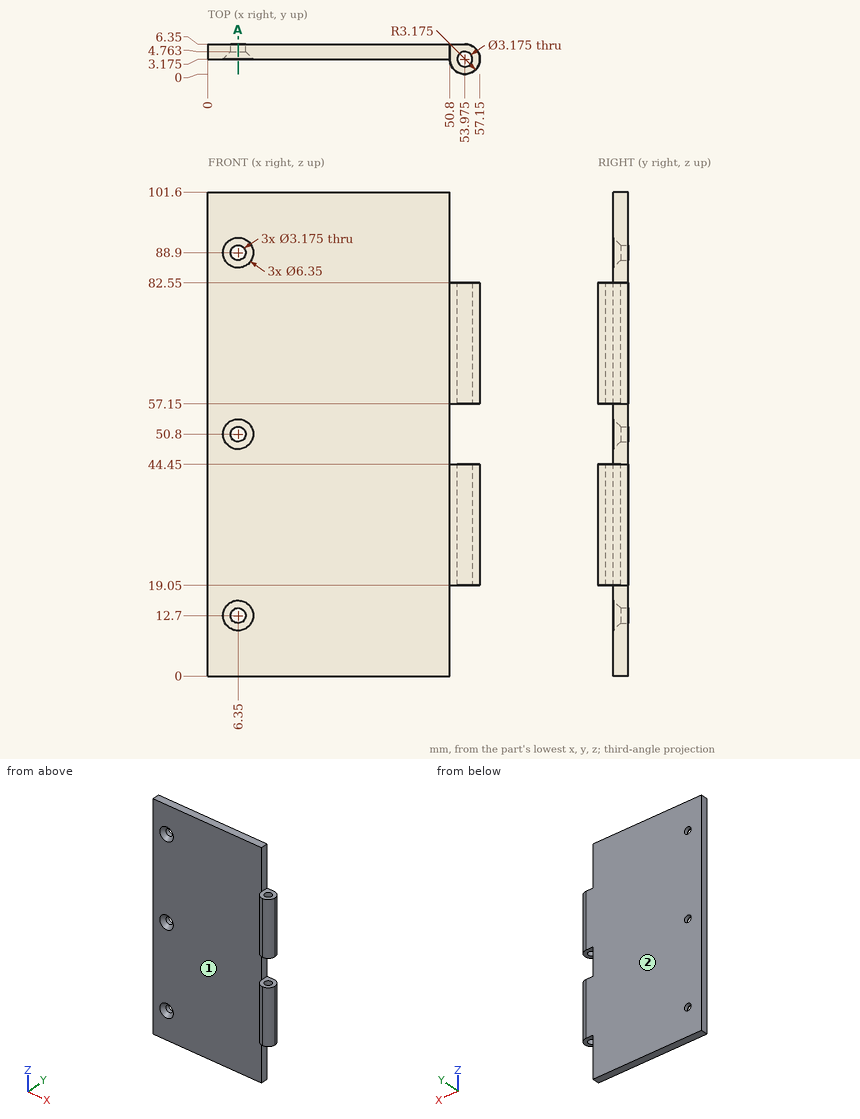
Geometry: see drawing. Coordinates: mm, zero at the bounding-box minimum. A direction names the side the tool comes from. Round coordinates to 2 decimals unless told otherwise and drop trailing zeros. Write item = value, one per line. Start each with the question number.
(1) Set-up query: the marked faces 1 and 2. Return all of +Z, -Z, +X, -X, +Y, -Y with unobstructed straight access to the full face (end or side cutting, diameter ignored); none if empty.
(2) Section query A-A, the plane x = 6.35. State how many separate pieces and enclosed holes the cut face has, plus the area to 3 significant figures.
(3) Pin query (flat end, axial travel): pin 1 (2.5 mm diameter, centred on x = 6.35, z = 88.9, fed in from +Y); pin 2 (8 mm diameter, centred on x = 29, z = 38.5, fed in from -Y) (1 decimal); pin 3 (3 mm diameter, centred on x = 54, y = 3.5, fed in from +Z); pin 4 (3.5 mm diameter, centred on y = 4.5, z = 93.5, fed in from +X). Return the tip coordinate at first contact, or that it passes through.
(4) Ray query, line 1 along Z through (x, y) = (6.35, 6); line 2 along X through (y, z) = (5.7, 50.8); line 3 along X through (y, z) = (2, 23.5) (1 decimal). Return the intervals inside material, ascending. Write a range as from..to.
Conclusion:
q1.face_1 = +Z, -Z, -X, -Y
q1.face_2 = +Z, -Z, +X, -X, +Y
q2.separate_pieces = 4
q2.enclosed_holes = 0
q2.area = 285 mm2
q3.pin_1 = through
q3.pin_2 = 3.2
q3.pin_3 = 82.55
q3.pin_4 = 50.8
q4.line_1 = 0..11.11, 14.29..49.21, 52.39..87.31, 90.49..101.6
q4.line_2 = 0..4.76, 7.94..50.8
q4.line_3 = 51..52.9, 55..56.9
